Model file for the job. Use its own axes, mm. A direction names the side the tool comes from. Coordinates: 2 decimals unless noted, no trailing zeros. Write each loop counter-clockwise with the first axis right and the second up, starting at its lowest first coordinate (ties: lowest second). Pieces come first, ordered by that corner, then holes. Notation, with made-up numbers: M 72,21 L 125,21 A30 cw 125,57 Z; hole C 43.25,50.25 d7. An arc over 180 degrees is marked long. Put each result on its own line as item: value. Start each with the question number.
Q1. Which spindle directions (+Z, -Z, +X, -X, +Y, -Y) get a long thin tool onto all of the face, cutting with end or side? Do faces 5 (the flat face through (90, -10, 4)), 6 (the flat face through (89, 0, 1)). Say none if no direction does.
Q2. Drill centre lines: line 1 along X through (y, z) = (-10, 3); line 2 along Z through (x, y) = (51, -18); line 3 along Z through (x, y) = (58, -17.5). Where is each one in solid material? Low to high.
Q3. Cut at C-C (x = 11). Write the cut outline in (y, z).
Q4. Cut at A-A (x = 150). Write the cut outline in (y, z).
Q5. Drop flat-ended pins along their axis: pin 1 (5.5 mm diameter, centred on x = 150, y = -10, fed in from -Z); pin 2 (4 mm diameter, centred on x = 114, z = 6, fed in from -Y); pin 3 (11.5 mm diameter, centred on x = 30, y = -10, fed in from +Z). Give the stop position or say it passes through.
Q6. Pull direction X, two halves, no side cores. Call faces 1 (the flat face through (180, -12, 12)), 2 (the flat face through (0, -12, 12)), 3 (the cylindrical face through (94.46, -10.59, 1.97)), 4 (the cylindrical face through (26.01, -7.92, 1.97)): pulls with the +X half, pulls with the -X half, needs draft (parallel to the pull), parting line crosses it, or undercut.
Q7. Cut at B-B (y = -10). Write the cut outline in (x, z).
Q8. Cut at D-D (z = 23). Write the cut outline in (x, y).
```python
from build123d import *

# Parameters (mm, degrees)
PAD_DEPTH            = 180
SKETCH001_R          = 4.5
POCKET_DEPTH         = 4
LINEARPATTERN_COUNT  = 3
LINEARPATTERN_PITCH  = 60
BODY_PLACEMENT_ANGLE = 90


with BuildPart() as part:
    # Sketch → Pad (new body)
    with BuildSketch(Plane.YZ):
        with BuildLine():
            Line((0, 30), (0, 0))
            Line((0, 0), (3, 0))
            ThreePointArc((3, 0), (19.18792, 4.611843), (30.514835, 17.0625))
            Line((29.124298, 18.5), (30.514835, 17.0625))
            ThreePointArc((2, 30), (11.754552, 15.269271), (29.124298, 18.5))
            Line((0, 30), (2, 30))
        make_face()
    extrude(amount=PAD_DEPTH)

    # Sketch001 (on Face1 of Pad) → Pocket (cut)
    with BuildSketch(Plane(origin=(0, 0, 0), x_dir=(0, 0, -1), z_dir=(0, -1, 0))):
        with Locations((-10, 30)):
            Circle(SKETCH001_R)
    pocket = extrude(amount=-POCKET_DEPTH, mode=Mode.SUBTRACT)

    # LinearPattern: Pocket ×3
    with Locations(*[(i * LINEARPATTERN_PITCH, 0, 0) for i in range(1, LINEARPATTERN_COUNT)]):
        add(pocket, mode=Mode.SUBTRACT)


with BuildPart() as part_1:
    # Body placement: moved
    add(part.part.rotate(Axis((0, 0, 0), (1, 0, 0)), BODY_PLACEMENT_ANGLE))


solid = part_1.part
```
Computed values:
1. face 5: -Z
1. face 6: +Z, -Z, +X, -X, +Y
2. line 1: 0 to 25.5, 34.5 to 85.5, 94.5 to 145.5, 154.5 to 180
2. line 2: 0 to 7.42, 28.58 to 29.61
2. line 3: 0 to 8.01, 27.99 to 30.09
3. outline: M -30,0 L 0,0 L 0,3 A30.72 ccw -17.06,30.51 L -18.5,29.12 A16 cw -30,2 Z
4. outline: M -30,0 L -14.5,0 L -14.5,4 L -5.5,4 L -5.5,0 L 0,0 L 0,3 A30.72 ccw -17.06,30.51 L -18.5,29.12 A16 cw -30,2 Z
5. pin 1: z = 4
5. pin 2: y = -22.25
5. pin 3: z = 29.82
6. face 1: pulls with the +X half
6. face 2: pulls with the -X half
6. face 3: undercut
6. face 4: undercut
7. outline: M 0,0 L 25.5,0 L 25.5,4 L 34.5,4 L 34.5,0 L 85.5,0 L 85.5,4 L 94.5,4 L 94.5,0 L 145.5,0 L 145.5,4 L 154.5,4 L 154.5,0 L 180,0 L 180,25.68 L 0,25.68 Z
8. outline: M 0,-14.8 L 180,-14.8 L 180,-7.4 L 0,-7.4 Z
